Design review of the part built by this model. Coordinates are the model's own, in mm. A direction names the side the tool comes from. Round coordinates to 2 decimals unless told otherwise and drop trailing zeros. Order: outer loops, then holes, each group sorted by start corner. A loop starts at its lowest first (then second) coordinate and runs counter-clockwise, first axis right, second up. Notation, with made-up numbers: (36.5, -11.75) - (58.5, -11.75) arc R29 cw to (58.5, 26.25) - close; hole circle Ø9 at (25.5, -6). An arc over 180 degrees is marked (long way). Write item = value, one per line.
from build123d import *

# Parameters (mm, degrees)
SKETCH10_R          = 3.175
BOSS_EXTRUDE4_DEPTH = 10
SKETCH11_R          = 15
BOSS_EXTRUDE5_DEPTH = 20
SKETCH12_R          = 2.85
CUT_EXTRUDE4_DEPTH  = 37
SKETCH13_R          = 6
CUT_EXTRUDE5_DEPTH  = 5
CHAMFER2_SIZE       = 1


with BuildPart() as part:
    # Sketch10 → Boss-Extrude4 (new body)
    with BuildSketch(Plane(origin=(0, 0, 0), x_dir=(1, 0, 0), z_dir=(0, 1, 0))):
        with BuildLine():
            Line((-40.573129599, -74.934887896), (0, -107.71591519))
            Line((0, -107.71591519), (40.573129599, -74.934887896))
            ThreePointArc((40.573129599, -74.934887896), (61.667652482, -77.175669978), (59.426870401, -98.270192861))
            Line((59.426870401, -98.270192861), (9.426870401, -138.667652482))
            ThreePointArc((9.426870401, -138.667652482), (0, -142), (-9.426870401, -138.667652482))
            Line((-9.426870401, -138.667652482), (-59.426870401, -98.270192861))
            ThreePointArc((-59.426870401, -98.270192861), (-61.667652482, -77.175669978), (-40.573129599, -74.934887896))
        make_face()
        with Locations((0, -127)):
            Circle(SKETCH10_R, mode=Mode.SUBTRACT)
    extrude(amount=BOSS_EXTRUDE4_DEPTH)

    # Sketch11 → Boss-Extrude5 (add)
    with BuildSketch(Plane(origin=(0, 10, 0), x_dir=(1, 0, 0), z_dir=(0, 1, 0))):
        with Locations((-50, -86.602540378)):
            Circle(SKETCH11_R)
        with Locations((50, -86.602540378)):
            Circle(SKETCH11_R)
    extrude(amount=BOSS_EXTRUDE5_DEPTH)

    # Sketch12 → Cut-Extrude4 (cut)
    with BuildSketch(Plane(origin=(0, 30, 0), x_dir=(1, 0, 0), z_dir=(0, 1, 0))):
        with Locations((-50, -86.602540378)):
            Circle(SKETCH12_R)
        with Locations((50, -86.602540378)):
            Circle(SKETCH12_R)
    extrude(amount=-CUT_EXTRUDE4_DEPTH, mode=Mode.SUBTRACT)

    # Sketch13 → Cut-Extrude5 (cut)
    with BuildSketch(Plane(origin=(0, 10, 0), x_dir=(1, 0, 0), z_dir=(0, 1, 0))):
        with Locations((0, -127)):
            Circle(SKETCH13_R)
    extrude(amount=-CUT_EXTRUDE5_DEPTH, mode=Mode.SUBTRACT)

    # Chamfer2
    chamfer2_edges = [part.edges().sort_by_distance(p)[0] for p in [
        (-52.85, 30, 86.602540378),
        (47.15, 30, 86.602540378),
        (-6, 10, 127),
    ]]
    chamfer(chamfer2_edges, length=CHAMFER2_SIZE)


solid = part.part
1) Clearance check with flat-ended pins moving along their axes: pin 1 Ø19 at (x, z) = (0, 127) entering from +Y; pin 2 Ø1 at (x, y) = (9.5, 10) entering from -Z; pin 3 Ø5 at (x, y) = (7, 6) entering from +Z. State where each tip first meets the part, or that it passes through.
Findings:
pin_1 = 10
pin_2 = 99.64
pin_3 = 141.31
2) To check wall thickness, follow L1, parallel to X at y = 16, z = 86; L2, parallel to Y at x = -31, z = 107; L3, parallel to X at y = 24, z = 90.5. State the ranges of each line that lie inside material, in increasing order. Write a range as from..to.
Findings:
L1 = -64.99..-52.79, -47.21..-35.01, 35.01..47.21, 52.79..64.99
L2 = 0..10
L3 = -64.48..-35.52, 35.52..64.48
3) The part is to be moulded in two halves that separate along Z. For faces 4 (the flat face through (34.777, 4.93, 118.186)), 5 (the cylindrical face through (49.382, 14.703, 89.385)), 6 (the flat face through (-47, 30, 90)), say which applies: released by +Z, released by -Z, zero draft, split by the parting line, or undercut.
Findings:
face_4 = released by +Z
face_5 = undercut
face_6 = zero draft
4) For faces 1 (the flat face through (3, 5, 130)), 2 (the flat face through (-20.571, 4.93, 91.096)), 3 (the cylindrical face through (-0.41, 2.46, 123.85)), list the 3-axis set-ups (+Z, -Z, +X, -X, +Y, -Y) from which the entire face can be reached by the end or side of a thin tool; tool diameter is ignored.
Findings:
face_1 = +Y
face_2 = -Z, +Y, -Y
face_3 = +Y, -Y
5) We need section A-A on z = 103. Write out the cut boundary in (x, y).
Findings:
outline = (-53.57, 0) - (-5.84, 0) - (-5.84, 10) - (-53.57, 10) - close; (5.84, 0) - (53.57, 0) - (53.57, 10) - (5.84, 10) - close
6) We need section C-C on y = 23.75. Write out the cut boundary in (x, z).
Findings:
outline = circle Ø30 at (-50, 86.6); circle Ø30 at (50, 86.6); hole circle Ø5.7 at (-50, 86.6); hole circle Ø5.7 at (50, 86.6)
7) We need section D-D on x = 42.5. Write out the cut boundary in (y, z).
Findings:
outline = (0, 73.61) - (30, 73.61) - (30, 99.59) - (10, 99.59) - (10, 111.95) - (0, 111.95) - close
8) We need section B-B on x = -50. Write out the cut boundary in (y, z).
Findings:
outline = (0, 71.6) - (30, 71.6) - (30, 82.75) - (29, 83.75) - (0, 83.75) - close; (0, 89.45) - (29, 89.45) - (30, 90.45) - (30, 101.6) - (10, 101.6) - (10, 105.89) - (0, 105.89) - close
